from build123d import *

# Parameters (mm, degrees)
F2_R            = 13.7514448946
F3_DEPTH        = 16
F5_DEPTH        = 16
F5_COPIES_COUNT = 18
F8_R            = 16.2514448946
F8_R_2          = 13.7514448946
F9_DEPTH        = 1.5
F10_DEPTH       = 17.501


# Not quite as in the source:
# - a feature of the source that left no trace in its solid (it failed there, or was rolled back) is left out
# - a pattern or mirror of a feature is missing from the dataset's text; its kind, count and spacing are read off the source's solid


with BuildPart() as f3:
    # F2 (on Top) → F3 (new body)
    with BuildSketch(Plane.XY):
        Circle(F2_R)
    extrude(amount=F3_DEPTH)

    # F4 (on face) → F5 (cut, through all)
    with BuildSketch(Plane.XY.offset(16)):
        with BuildLine():
            ThreePointArc((-2.015669756, 13.6029155744), (-1.6587079327, 13.5010225766), (-1.499776395, 13.1655457628))
            ThreePointArc((-1.499776395, 13.1655457628), (0, 11.6914448946), (1.499776395, 13.1655457628))
            ThreePointArc((1.499776395, 13.1655457628), (1.6587079327, 13.5010225766), (2.015669756, 13.6029155744))
            ThreePointArc((2.015669756, 13.6029155744), (0, 13.7514448946), (-2.015669756, 13.6029155744))
        make_face()
    f5 = extrude(amount=-F5_DEPTH, mode=Mode.SUBTRACT)

    # F5_copies: F5 ×18 about axis
    f5_copies_axis = Axis((0, 0, 0), (0, 0, 1))
    for i in range(1, F5_COPIES_COUNT):
        add(f5.rotate(f5_copies_axis, i * 360 / F5_COPIES_COUNT), mode=Mode.SUBTRACT)

    # F8 (on face) + F2 (on Top) → F9 (join)
    with BuildSketch(Plane.XY):
        Circle(F8_R)
        Circle(F8_R_2, mode=Mode.SUBTRACT)
    with BuildSketch(Plane.XY):
        Circle(F2_R)
    extrude(amount=-F9_DEPTH)

    # F7 (on face) → F10 (cut, through all)
    with BuildSketch(Plane.XY.offset(16)):
        Polygon((3.7527767497, 6.5), (-3.7527767497, 6.5), (-7.5055534995, 0), (-3.7527767497, -6.5), (3.7527767497, -6.5), (7.5055534995, 0), align=None)
    extrude(amount=-F10_DEPTH, mode=Mode.SUBTRACT)


solid = f3.part
Model file for the job. Use its own axes, mm. A direction names the side the tool comes from. Give positions to 0.01 mm unless a question says otherwise; leave off trailing zeros. Order: outer loops, then holes, each group sorted by start corner. A loop starts at its lowest first (then second) coordinate and runs counter-clockwise, first axis right, second up. Notation, with made-up numbers: M -7,22 L 37,22 A12 cw 37,28 Z; hole C 5,73 d7. An arc over 180 degrees is marked long. Write item = value, one per line.
Q1. Tool access for faces 3 (the cylindrical face through (10.11, 5.87, 8.11)), 4 (the flat face through (-6, -3, 16)), 5 (the flat face through (5.6, -3.3, 7.4)), 6 (the cylindrical face through (-0.03, 11.69, 8.11)): list every direction of +Z, -Z, +X, -X, +Y, -Y with a clear straight run to the whole face (end or side of a thin tool).
Derived:
face_3 = +Z
face_4 = +Z, +X, -X, +Y, -Y
face_5 = +Z, -Z
face_6 = +Z, +Y
Q2. Flat gauge pins, fed straight in: pin 1 (6 mm diameter, centred on y = -3.5, z = 12, fed in from +X); pin 2 (6 mm diameter, centred on x = -9, z = 7, fed in from -Y); pin 3 (1.5 mm diameter, centred on x = 7.5, z = 0.5, fed in from -Y). Where does each tip first touch, or does it go through?
Derived:
pin_1 = 13.73
pin_2 = -12.15
pin_3 = -14.69
Q3. Cut at C-C, the plane y = -10. List the corners of the cut face in (x, z), then the cut area to 3 significant figures.
Derived:
outline = M -12.81,-1.5 L 12.81,-1.5 L 12.81,0 L 6.98,0 L 6.98,16 L -6.98,16 L -6.98,0 L -12.81,0 Z
area = 262 mm2
Q4. Two-plate mould, pull along X, no slides. Class faces 1 (the cylindrical face through (0.03, -11.69, 8.11)), 2 (the flat face through (0, -7, -1.5)): pulls with the +X half, pulls with the -X half, needs draft (parallel to the pull), parting line crosses it, or undercut.
Derived:
face_1 = undercut
face_2 = needs draft
Q5. Cut at A-A, the plane x = 0. List the corners of the cut face in (y, z), then the cut area to 3 significant figures.
Derived:
outline = M -16.25,-1.5 L -6.5,-1.5 L -6.5,16 L -11.69,16 L -11.69,0 L -16.25,0 Z; M 6.5,-1.5 L 16.25,-1.5 L 16.25,0 L 11.69,0 L 11.69,16 L 6.5,16 Z
area = 195 mm2
Q6. Cut at B-B, the plane x = 8. List the corners of the cut face in (y, z), then the cut area to 3 significant figures.
Derived:
outline = M -14.15,-1.5 L 14.15,-1.5 L 14.15,0 L 8.68,0 L 8.68,16 L -8.68,16 L -8.68,0 L -14.15,0 Z
area = 320 mm2
Q7. Drill centre lines: line 1 (X direction, y = -9, z = 0.75); line 2 (Y direction, x = 12, z = 9.5); line 3 (Z direction, x = -13.5, y = 2). Where is each one in solid material? Low to high. Write a range as [from, to].
Derived:
line_1 = [-10.4, -9.49], [-7.47, 7.47], [9.49, 10.4]
line_2 = [-5.21, -3.42], [-1.16, 1.16], [3.42, 5.21]
line_3 = [-1.5, 0]
